Verification items for the finished model (mm, model axes). Round coordinates to 2 decimals unless told otherwise and drop trailing zeros. Write each loop counter-clockwise with the first axis right and the second up, starting at its lowest first coordinate (ties: lowest second). Pieces come first, ordered by that corner, then holes. Notation, with made-up numbers: (0, 64) -> (10, 64) arc R20 ccw to (10, 73) -> close; hole circle Ø9 at (-28.75, 10.25). An arc over 180 degrees is marked (long way). Answer as a JSON object with one key per item and string values. Group by question number.
(1) Sectioned sample at A-A on x = -7. Record the cut outline in (y, z), and give its area (3 significant figures).
(2) Sectioned sample at D-D on z = 96. Record the cut outline in (x, y), and give its area (3 significant figures).
(3) Sectioned sample at B-B on x = 0. Record the cut outline in (y, z).
(4) Scan lines: L1, parallel to Z at x = 7.25, y = -2.75; L2, parallel to X at y = 0.25, z = 84; L3, parallel to X at y = -8, z = 88.5. Record each from-to range of solid material in increasing order. Write a range as from..to.
(5) Gauge pin test, flat ends, axial feed: pin 1 Ø6 at (x, z) = (6, 39.5) entering from -Y; pin 2 Ø1.5 at (y, z) = (-6.5, 79) entering from -X; pin 3 Ø1 at (y, z) = (1, 100.5) entering from +X. Record the tip position at first contact, or that the pin passes through.
```python
from build123d import *

# Parameters (mm, degrees)
F0_R     = 9
F1_DEPTH = 120
F2_R     = 5
F3_DEPTH = 5
F4_R     = 9
F4_R_2   = 5
F5_DEPTH = 5
F6_R     = 5
F7_DEPTH = 5
F8_R     = 9
F8_R_2   = 5
F9_DEPTH = 5


with BuildPart() as f1:
    # F0 (on Top) → F1 (new body)
    with BuildSketch(Plane.XY):
        Circle(F0_R)
    extrude(amount=F1_DEPTH)

    # F2 (on face) → F3 (join)
    with BuildSketch(Plane.XY.offset(120)):
        Circle(F2_R)
    extrude(amount=F3_DEPTH)

    # F4 (on face) → F5 (join)
    with BuildSketch(Plane.XY.offset(125)):
        Circle(F4_R)
        Circle(F4_R_2, mode=Mode.SUBTRACT)
        Circle(F4_R_2)
    extrude(amount=F5_DEPTH)

    # F6 (on face) → F7 (join)
    with BuildSketch(Plane(origin=(0, 0, 0), x_dir=(1, 0, 0), z_dir=(0, 0, -1))):
        Circle(F6_R)
    extrude(amount=F7_DEPTH)

    # F8 (on face) → F9 (join)
    with BuildSketch(Plane(origin=(0, 0, -5), x_dir=(1, 0, 0), z_dir=(0, 0, -1))):
        Circle(F8_R)
        Circle(F8_R_2, mode=Mode.SUBTRACT)
        Circle(F8_R_2)
    extrude(amount=F9_DEPTH)


solid = f1.part
```
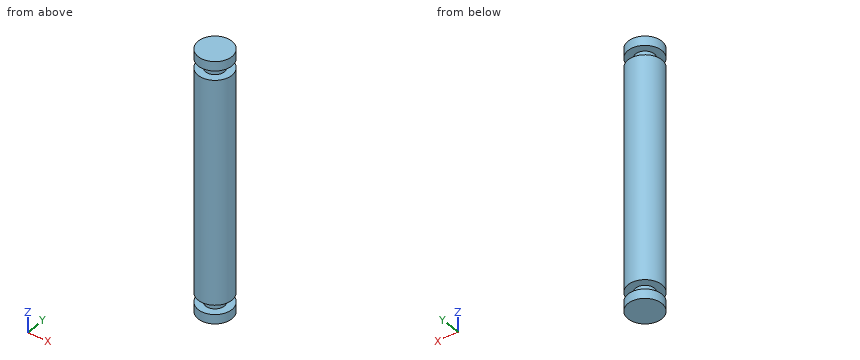
Computed values:
{
 "1": {"outline": "(-5.66, -10) -> (5.66, -10) -> (5.66, -5) -> (-5.66, -5) -> close; (-5.66, 0) -> (5.66, 0) -> (5.66, 120) -> (-5.66, 120) -> close; (-5.66, 125) -> (5.66, 125) -> (5.66, 130) -> (-5.66, 130) -> close", "area": "1,470 mm2"},
 "2": {"outline": "circle Ø18 at (0, 0)", "area": "254 mm2"},
 "3": {"outline": "(-9, -10) -> (9, -10) -> (9, -5) -> (5, -5) -> (5, 0) -> (9, 0) -> (9, 120) -> (5, 120) -> (5, 125) -> (9, 125) -> (9, 130) -> (-9, 130) -> (-9, 125) -> (-5, 125) -> (-5, 120) -> (-9, 120) -> (-9, 0) -> (-5, 0) -> (-5, -5) -> (-9, -5) -> close"},
 "4": {"L1": "-10..-5, 0..120, 125..130", "L2": "-9..9", "L3": "-4.12..4.12"},
 "5": {"pin 1": "y = -8.49", "pin 2": "x = -6.92", "pin 3": "x = 8.99"}
}
